Can you work these out from the model? Positions are in its coordinate system, mm. A direction names the side the tool comes from. Round coordinates to 2 decimals unless told otherwise and drop trailing zeros. Write each loop counter-clockwise with the first axis right and the second up, starting at its lowest first coordinate (ties: lowest second). Pieces come first, ordered by that corner, then holes. Notation, with made-up numbers: M -35.5,-36 L -14.5,-36 A13 cw -14.5,-16 Z; hole C 52.5,21.5 d8. An arc over 180 degrees is marked long. Answer in a Markdown table with one row per item. Add a question column.
(1) If I drill on probe 1 along X at (y, z) = (-4, 81) (3 decimals); probe 2 along Y at (x, z) = (-0.25, 126); probe 3 along Y at (x, z) = (-5.5, 62.5), over which ranges is the centre line in solid material (lowest first)?
(2) If we mould it in two halves opening along X, with no side actions, what happens to faces 1 (the face through (-10.795, 0, 69)), 2 (the face through (-0.148, -17.806, 69.194)), 3 (the face through (9.081, 1.705, 4.443))? For each: released by +X, released by -X, zero draft, split by the parting line, or undercut.
(3) I'm going to push flat-ended pins straight in: pin 1 (6 mm diameter, centred on x = 8.5, z = 117, fed in from +Y); pin 2 (8 mm diameter, centred on x = 8, z = 93.5, fed in from -Y). Where does each tip first touch, or does it pass through?
(4) Suppose I cut it at A-A, the plane z = 17. Write out the boundary of the cut face in (x, y) (3 decimals).
(5) For faces 4 (the face through (-8.89, 0, 69)), 5 (the face through (-10.6, 1.54, 4.38)), which set-ups out of +Z, -Z, +X, -X, +Y, -Y let a thin tool reach every point of the face, with its end or its side?
from build123d import *

# Parameters (mm, degrees)
F1_DEPTH = 139.7
F3_DEPTH = 10.795
F4_R     = 0.635


with BuildPart() as f1:
    # F0 (on Top) → F1 (new body)
    with BuildSketch(Plane.XY):
        with BuildLine():
            Line((-9.965403, 14.724749), (-10.795, 13.15232))
            Line((-10.795, 13.15232), (-10.795, -13.15232))
            Line((-10.795, -13.15232), (-9.965403, -14.724749))
            ThreePointArc((-9.965403, -14.724749), (0, -17.806574), (9.965403, -14.724749))
            Line((9.965403, -14.724749), (10.795, -13.15232))
            Line((10.795, -13.15232), (10.795, 13.15232))
            Line((10.795, 13.15232), (9.965403, 14.724749))
            ThreePointArc((9.965403, 14.724749), (0, 17.806574), (-9.965403, 14.724749))
        make_face()
        with BuildLine():
            Line((-8.89, -13.15232), (-8.89, 13.15232))
            ThreePointArc((-8.89, 13.15232), (0, 15.901574), (8.89, 13.15232))
            Line((8.89, 13.15232), (8.89, -13.15232))
            ThreePointArc((8.89, -13.15232), (0, -15.901574), (-8.89, -13.15232))
        make_face(mode=Mode.SUBTRACT)
    extrude(amount=F1_DEPTH)

    # F2 (on Right) → F3 (cut, symmetric)
    with BuildSketch(Plane.YZ):
        Polygon((24.65296, 12.700437), (-9.836838, 0), (0, 0), (24.65296, 0), align=None)
    extrude(amount=F3_DEPTH, both=True, mode=Mode.SUBTRACT)

    # F4
    f4_edges = [f1.edges().sort_by_distance(p)[0] for p in [
        (10.795, 1.657741, 4.232735),
        (0, 17.806574, 10.179341),
        (0, 15.901574, 9.477848),
        (8.89, 1.657741, 4.232735),
        (-10.795, 1.657741, 4.232735),
        (10.380202, 13.938535, 8.754984),
        (-10.380202, 13.938535, 8.754984),
        (-10.795, -11.494579, 0),
        (-10.380202, -13.938535, 0),
        (0, -17.806574, 0),
        (0, -15.901574, 0),
        (8.89, -11.494579, 0),
        (10.795, -11.494579, 0),
        (10.380202, -13.938535, 0),
        (-8.89, -11.494579, 0),
        (-8.89, 1.657741, 4.232735),
    ]]
    fillet(f4_edges, radius=F4_R)


solid = f1.part
Calculated:
| question | item | result |
|---|---|---|
| 1 | probe 1 | -10.795 to -8.89, 8.89 to 10.795 |
| 1 | probe 2 | -17.8 to -15.9, 15.9 to 17.8 |
| 1 | probe 3 | -16.93 to -14.91, 14.91 to 16.93 |
| 2 | face 1 | released by -X |
| 2 | face 2 | split by the parting line |
| 2 | face 3 | undercut |
| 3 | pin 1 | y = 16.93 |
| 3 | pin 2 | y = -17.35 |
| 4 | outline | M -10.795,-13.152 L -9.965,-14.725 A17.653 ccw 9.965,-14.725 L 10.795,-13.152 L 10.795,13.152 L 9.965,14.725 A17.653 ccw -9.965,14.725 L -10.795,13.152 Z; hole M -8.89,-13.152 A15.748 ccw 8.89,-13.152 L 8.89,13.152 A15.748 ccw -8.89,13.152 Z |
| 5 | face 4 | +Z, -Z |
| 5 | face 5 | -Z, -X, +Y |
